Verification items for the finished model (mm, model axes). A direction names the side the tool comes from. Round coordinates to 2 decimals unless told otherwise and drop trailing zeros. Write each loop counter-clockwise with the first axis right and the second up, starting at its lowest first coordinate (ties: lowest second). Pieces come first, ordered by that corner, then holes. Notation, with made-up numbers: (-19.5, 12) -> (36.5, 12) arc R12 ccw to (36.5, 35) -> close; hole circle Ø4 at (78.25, 9). An arc over 180 degrees is marked (long way). Answer as a JSON object with one key per item and string values. Group by question number.
(1) Draft check along X on faces 4 (the face through (-70, 0, 22)), 5 (the face through (-3.23, 60.79, -0.21)), 6 (the face through (-14, 45, -5)). Enter one of: released by +X, released by -X, zero draft, split by the parting line, or undercut.
(2) Sectioned sample at D-D on x = -11.5. Record the cut outline in (y, z).
(3) Sectioned sample at C-C on z = 9. Record the cut outline in (x, y), and give its area (3 significant figures).
(4) Gauge pin test, flat ends, axial feed: pin 1 Ø4 at (x, z) = (-62, -19) entering from +Y; pin 2 Ø20.5 at (y, z) = (48, 0) entering from +X; pin 3 Ø6 at (y, z) = (73, 20) entering from +X; pin 4 Ø15.5 at (y, z) = (42.5, 13.5) entering from +X. Record the tip position at first contact, or that the pin passes through.
(5) Scan lines: L1, parallel to Y at x = 0, z = 3; L2, parallel to Y at x = -17, z = 22.5; L3, parallel to X at y = 70.5, z = 12. Record each from-to range of solid material in increasing order. Write a range as from..to.
(6) Sectioned sample at B-B on y = 48. Record the cut outline in (x, z), and give its area (3 significant figures).
(7) Set-up check for faces 1 (the face through (14, 45, -5)), 2 (the face through (-14.51, 36.51, 0.51)), 3 (the face through (70, 2, -17)): record each of +Z, -Z, +X, -X, +Y, -Y from which the full face is reachable in a straight line by a thin tool's end or side.
(8) Sectioned sample at A-A on x = 58. Record the cut outline in (y, z), and give its area (3 significant figures).
```python
from build123d import *

# Parameters (mm, degrees)
SKETCH_1_W                  = 160
SKETCH_1_H                  = 56
EXTRUDE_1_DEPTH             = 16
SKETCH_2_W                  = 160
SKETCH_2_H                  = 34
CUT_EXTRUDE_1_DEPTH         = 4
SKETCH_3_W                  = 120
SKETCH_3_H                  = 56
CUT_EXTRUDE_2_DEPTH         = 4
EXTRUDE_2_DEPTH             = 2
EXTRUDE_3_DEPTH             = 15
CUT_EXTRUDE_START           = -30
CUT_EXTRUDE_3_DEPTH         = 30
HOLE_WIZARD_M16_1_D         = 14
HOLE_WIZARD_M6_1_REACH      = 119.932
HOLE_WIZARD_M6_1_BORE_R     = 2.5
HOLE_START                  = -15
HOLE_WIZARD_1_OUTLINE_R     = 5.5
HOLE_WIZARD_1_DEPTH         = 15
HOLE_WIZARD_1_2_OUTLINE_R   = 11.5
HOLE_WIZARD_1_2_OUTLINE_R_2 = 5.5
HOLE_WIZARD_1_2_DEPTH       = 1


# Read off the part's stored shape, not the designer's step: 切除-拉伸3, 孔1
with BuildPart() as part:
    # 草图1 → 凸台-拉伸1 (new body)
    with BuildSketch(Plane(origin=(0, 0, 0), x_dir=(1, 0, 0), z_dir=(0, 1, 0))):
        Rectangle(SKETCH_1_W, SKETCH_1_H)
    extrude(amount=EXTRUDE_1_DEPTH)

    # 草图2 → 切除-拉伸1 (cut)
    with BuildSketch(Plane.XZ):
        Rectangle(SKETCH_2_W, SKETCH_2_H)
    extrude(amount=-CUT_EXTRUDE_1_DEPTH, mode=Mode.SUBTRACT)

    # 草图3 → 切除-拉伸2 (cut)
    with BuildSketch(Plane.XZ):
        Rectangle(SKETCH_3_W, SKETCH_3_H)
    extrude(amount=-CUT_EXTRUDE_2_DEPTH, mode=Mode.SUBTRACT)

    # 草图4 → 凸台-拉伸2 (add)
    with BuildSketch(Plane(origin=(0, 16, 0), x_dir=(1, 0, 0), z_dir=(0, 1, 0))):
        with BuildLine():
            Line((-30, 11), (-80, 11))
            Line((-80, 11), (-80, 5))
            Line((-80, 5), (-30, 5))
            ThreePointArc((-30, 5), (-25, 0), (-30, -5))
            Line((-30, -5), (-80, -5))
            Line((-80, -5), (-80, -11))
            Line((-80, -11), (-30, -11))
            ThreePointArc((-30, -11), (-19, 0), (-30, 11))
        make_face()
    extrude_2 = extrude(amount=EXTRUDE_2_DEPTH)

    # 镜向1: 凸台-拉伸2 across plane
    add(extrude_2.mirror(Plane(origin=(0, 0, 0), x_dir=(0, 0, 1), z_dir=(1, 0, 0))))

    # 草图5 → 凸台-拉伸3 (add, symmetric)
    with BuildSketch(Plane(origin=(0, 0, 0), x_dir=(0, 0, -1), z_dir=(1, 0, 0))):
        Polygon((-28, 18), (-15, 50), (-15, 82), (15, 82), (15, 50), (28, 18), (28, 16), (-28, 16), align=None)
    extrude(amount=EXTRUDE_3_DEPTH, both=True)

    # 切除-拉伸3 outline → 切除-拉伸3 (cut)
    with BuildSketch(Plane.XY.offset(15).offset(CUT_EXTRUDE_START)):
        with BuildLine():
            Line((-15, 82), (-15, 67))
            ThreePointArc((-15, 67), (-10.606601718, 77.606601718), (0, 82))
            Line((0, 82), (-15, 82))
        make_face()
        with BuildLine():
            Line((15, 82), (0, 82))
            ThreePointArc((0, 82), (10.606601718, 77.606601718), (15, 67))
            Line((15, 67), (15, 82))
        make_face()
    extrude(amount=CUT_EXTRUDE_3_DEPTH, mode=Mode.SUBTRACT)

    # M16 螺纹孔1 (through all)
    with Locations(Plane.XY.offset(15)):
        with Locations((0, 67)):
            Hole(HOLE_WIZARD_M16_1_D / 2)

    # M6 螺纹孔1 bore → M6 螺纹孔1 (cut, up to next)
    with BuildSketch(Plane(origin=(0, 82, 0), x_dir=(1, 0, 0), z_dir=(0, 1, 0)), mode=Mode.PRIVATE) as hole_wizard_m6_1_sk1:
        Circle(HOLE_WIZARD_M6_1_BORE_R)
    hole_wizard_m6_1_tool1 = extrude(hole_wizard_m6_1_sk1.sketch, amount=-HOLE_WIZARD_M6_1_REACH, mode=Mode.PRIVATE) & part.part
    add(hole_wizard_m6_1_tool1.solids().sort_by_distance((0, 82, 0))[0], mode=Mode.SUBTRACT)

    # 孔1 outline → 孔1 (cut)
    with BuildSketch(Plane.YZ.offset(HOLE_START)):
        with Locations((48, 0)):
            Circle(HOLE_WIZARD_1_OUTLINE_R)
    hole_wizard_1 = extrude(amount=HOLE_WIZARD_1_DEPTH, mode=Mode.SUBTRACT)

    # Hole Wizard 1 2 outline → Hole Wizard 1 2 (cut)
    with BuildSketch(Plane.YZ.offset(HOLE_START)):
        with Locations((48, 0)):
            Circle(HOLE_WIZARD_1_2_OUTLINE_R)
        with Locations((48, 0)):
            Circle(HOLE_WIZARD_1_2_OUTLINE_R_2, mode=Mode.SUBTRACT)
    hole_wizard_1_2 = extrude(amount=HOLE_WIZARD_1_2_DEPTH, mode=Mode.SUBTRACT)

    # 镜向2: 孔1, Hole Wizard 1 2 across plane
    add(hole_wizard_1.mirror(Plane(origin=(0, 0, 0), x_dir=(0, 0, 1), z_dir=(1, 0, 0))), mode=Mode.SUBTRACT)
    add(hole_wizard_1_2.mirror(Plane(origin=(0, 0, 0), x_dir=(0, 0, 1), z_dir=(1, 0, 0))), mode=Mode.SUBTRACT)


solid = part.part
```
Computed values:
{
 "1": {"face 4": "zero draft", "face 5": "undercut", "face 6": "released by -X"},
 "2": {"outline": "(4, -28) -> (18, -28) -> (50, -15) -> (76.63, -15) -> (76.63, 15) -> (50, 15) -> (18, 28) -> (4, 28) -> close; hole circle Ø11 at (48, 0)"},
 "3": {"outline": "(-80, 4) -> (80, 4) -> (80, 18) -> (23.68, 18) -> (23.68, 16) -> (15, 16) -> (15, 40.84) -> (14, 40.84) -> (14, 55.16) -> (15, 55.16) -> (15, 67) arc R15 ccw to (-15, 67) -> (-15, 55.16) -> (-14, 55.16) -> (-14, 40.84) -> (-15, 40.84) -> (-15, 16) -> (-23.68, 16) -> (-23.68, 18) -> (-80, 18) -> close; hole circle Ø14 at (0, 67)", "area": "3,850 mm2"},
 "4": {"pin 1": "y = 16", "pin 2": "x = 14", "pin 3": "through", "pin 4": "x = 15"},
 "5": {"L1": "4..43.39, 52.61..60, 74..82", "L2": "4..16", "L3": "-14.59..-6.06, 6.06..14.59"},
 "6": {"outline": "(-15, -15.81) -> (15, -15.81) -> (15, -11.5) -> (14, -11.5) -> (14, -5.5) -> (-14, -5.5) -> (-14, -11.5) -> (-15, -11.5) -> close; (-15, 11.5) -> (-14, 11.5) -> (-14, 5.5) -> (14, 5.5) -> (14, 11.5) -> (15, 11.5) -> (15, 15.81) -> (-15, 15.81) -> close", "area": "595 mm2"},
 "7": {"face 1": "+X", "face 2": "-X", "face 3": "+X, -X, -Y"},
 "8": {"outline": "(4, -28) -> (16, -28) -> (16, -11) -> (18, -11) -> (18, -5) -> (16, -5) -> (16, 5) -> (18, 5) -> (18, 11) -> (16, 11) -> (16, 28) -> (4, 28) -> close", "area": "696 mm2"}
}
